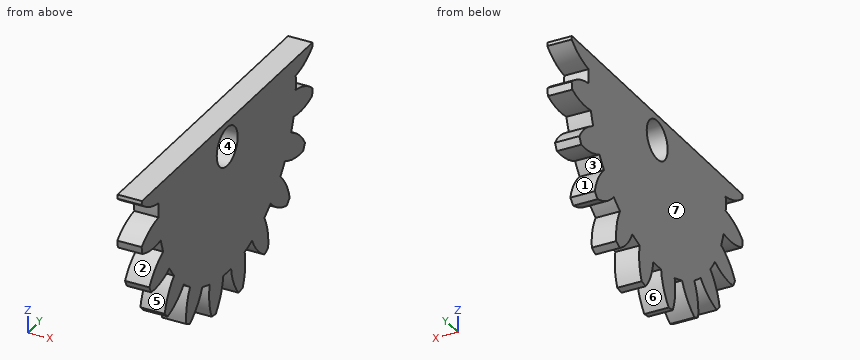
```python
from build123d import *

# Parameters (mm, degrees)
BASPROSKE_W        = 2.5
BASPROSKE_H        = 16.5
TOOTHCUT_DEPTH     = 24.468063405
TEETHCUTS_COUNT    = 20
TEETHCUTS_ANGLE    = 342
BORSKE_R           = 2
BORE_DEPTH         = 50.0000508
SKETCH1_W          = 14.029900708
SKETCH1_H          = 46.240429445
CUT_EXTRUDE1_DEPTH = 24.26283946


with BuildPart() as part:
    # BasProSke → Base-Revolve (revolve)
    with BuildSketch(Plane(origin=(0, 0, 0), x_dir=(1, 0, 0), z_dir=(0, 1, 0)), mode=Mode.PRIVATE) as base_revolve_sk:
        with Locations((1.25, 8.25)):
            Rectangle(BASPROSKE_W, BASPROSKE_H)
    revolve(base_revolve_sk.sketch.rotate(Axis((-10, 0, 0), (1, 0, 0)), 180), axis=Axis((-10, 0, 0), (1, 0, 0)))

    # TooCutSke → ToothCut (cut, through all)
    with BuildSketch(Plane(origin=(0, 0, 0), x_dir=(0, 0, -1), z_dir=(1, 0, 0))):
        with BuildLine():
            ThreePointArc((0.74381438, 13.102904875), (0, 13.124), (-0.74381438, 13.102904875))
            ThreePointArc((-0.74381438, 13.102904875), (-1.226473103, 14.852072512), (-2.209965745, 16.376962373))
            ThreePointArc((-2.209965745, 16.376962373), (0, 16.5254), (2.209965745, 16.376962373))
            ThreePointArc((2.209965745, 16.376962373), (1.226473103, 14.852072512), (0.74381438, 13.102904875))
        make_face()
    toothcut = extrude(amount=TOOTHCUT_DEPTH, mode=Mode.SUBTRACT)

    # TeethCuts: ToothCut ×20 about axis
    teethcuts_axis = Axis((-10, 0, 0), (1, 0, 0))
    for i in range(1, TEETHCUTS_COUNT):
        add(toothcut.rotate(teethcuts_axis, i * TEETHCUTS_ANGLE / (TEETHCUTS_COUNT - 1)), mode=Mode.SUBTRACT)

    # BorSke → Bore (cut, symmetric)
    with BuildSketch(Plane(origin=(0, 0, 0), x_dir=(0, 0, -1), z_dir=(1, 0, 0))):
        with Locations(Location((0, 0, 0), (0, 0, 180))):
            Circle(BORSKE_R)
    extrude(amount=BORE_DEPTH, both=True, mode=Mode.SUBTRACT)

    # Sketch1 → Cut-Extrude1 (cut, through all)
    with BuildSketch(Plane(origin=(2.5, 0, 0), x_dir=(0, 0, -1), z_dir=(1, 0, 0))):
        with Locations((-9.596119027, 6.823357103)):
            Rectangle(SKETCH1_W, SKETCH1_H)
    extrude(amount=-CUT_EXTRUDE1_DEPTH, mode=Mode.SUBTRACT)


solid = part.part
```
CAD build for the part. Positions are in the model's coordinates, mm. Face numbers are marked on the shaded views. A direction names the side the tool comes from. Round coordinates to 2 decimals unless told otherwise and drop trailing zeros. Write each loop counter-clockwise with the first axis right and the second up, starting at its lowest first coordinate (ties: lowest second). Pieces come first, ordered by that corner, then holes. Notation, with made-up numbers: (-33.75, 71.25) -> (-2.75, 71.25) arc R25 ccw to (-2.75, 94.25) -> close; hole circle Ø5 at (49.25, 21.5). An arc over 180 degrees is marked (long way). Answer in a Markdown table with one row per item. Add a question column.
Item 1: Which spindle directions (+Z, -Z, +X, -X, +Y, -Y) get a long thin tool onto all of the face, cutting with end or side? Do the marked faces 1, 2 and 3. Say none if no direction does.
Item 2: Saw through at C-C, the plane z = -10.5. Write the cut outline in (x, y), then the cut area to 3 significant figures.
Item 3: Drill centre lines: line 1 (Y direction, x = 0.9, z = -13); line 2 (Y direction, x = 0.75, z = 0); line 3 (Y direction, x = 2.2, z = -11.5). Where is each one in solid material? Low to high. Write a range as from..to.
Item 4: Mould opens along Y. For the marked faces 4, 5, 6 and 7 say: pulls with the +Y half, pulls with the -Y half, needs draft (parallel to the pull), parting line crosses it, or undercut.
Item 5: Drop flat-ended pins along their axis: pin 1 Ø4 at (y, z) = (-1, -7) entering from -X; pin 2 Ø1.5 at (x, z) = (0.5, -6) entering from -Y. Give the stop position or say it passes through.
Item 6: Saw through at D-D, the plane y = 4. Write the cut outline in (x, z).
Item 7: Saw through at A-A, the plane z = 0. Write the cut outline in (x, y).
Item 8: Saw through at B-B, the plane y = 0. Write the cut outline in (x, z).
Findings below:
| question | item | result |
|---|---|---|
| 1 | face 1 | +X, -X, +Y |
| 1 | face 2 | +X, -X, -Y |
| 1 | face 3 | +X, -X |
| 2 | outline | (0, -11.67) -> (2.5, -11.67) -> (2.5, -8.64) -> (0, -8.64) -> close; (0, -7.87) -> (2.5, -7.87) -> (2.5, 7.87) -> (0, 7.87) -> close; (0, 8.64) -> (2.5, 8.64) -> (2.5, 11.67) -> (0, 11.67) -> close |
| 2 | area | 54.5 mm^2 |
| 3 | line 1 | y = -7.79..-5.18, -3.39..3.39, 5.18..7.79 |
| 3 | line 2 | y = -13.12..-2, 2..13.12 |
| 3 | line 3 | y = -11.83..-10.11, -7.33..7.33, 10.11..11.83 |
| 4 | face 4 | undercut |
| 4 | face 5 | pulls with the -Y half |
| 4 | face 6 | undercut |
| 4 | face 7 | needs draft |
| 5 | pin 1 | stops at x = 0 |
| 5 | pin 2 | stops at y = -14.63 |
| 6 | outline | (0, -12.5) -> (2.5, -12.5) -> (2.5, 2.58) -> (0, 2.58) -> close |
| 7 | outline | (0, -13.12) -> (2.5, -13.12) -> (2.5, -2) -> (0, -2) -> close; (0, 2) -> (2.5, 2) -> (2.5, 13.12) -> (0, 13.12) -> close |
| 8 | outline | (0, -13.12) -> (2.5, -13.12) -> (2.5, -2) -> (0, -2) -> close; (0, 2) -> (2.5, 2) -> (2.5, 2.58) -> (0, 2.58) -> close |
